```python
from build123d import *

# Parameters (mm, degrees)
F0_R     = 30
F1_DEPTH = 200
F5_START = 20
F4_R     = 45
F5_DEPTH = 30


with BuildPart() as f1:
    # F0 (on Right) → F1 (new body)
    with BuildSketch(Plane.YZ):
        Circle(F0_R)
    extrude(amount=-F1_DEPTH)

    # F2 (on Top) → F3 (revolve)
    with BuildSketch(Plane.XY):
        Polygon((0, 12.6511614473), (0, 0), (30.3976608496, 0), (30.3976608496, 8), align=None)
    revolve(axis=Axis((15.1988304248, 0, 0), (1, 0, 0)))

    # F4 (on Right) → F5 (join)
    with BuildSketch(Plane.YZ.offset(F5_START)):
        Circle(F4_R)
    extrude(amount=F5_DEPTH)


solid = f1.part
```
Read the model definition and answer for the solid it produces. Units are mm, in the model's axes. A direction names the side the tool comes from. Coordinates: 2 decimals unless noted, no trailing zeros. Loops run counter-clockwise (first coordinate to the right, second up) from the corner with the lowest first, then second, coordinate; pieces in that order, holes last.
(1) Consider line 1 along X through (y, z) = (25.5, 10); line 2 along X through (y, z) = (-4, -37.5); line 3 along Y through (x, z) = (-111, -0.5). Determine where each line is inside the solid, lowest interval first.
Solution:
line 1: x = -200 to 0, 20 to 50
line 2: x = 20 to 50
line 3: y = -30 to 30
(2) The part is cut by section A-A (y = 25). Determine the outline of the cut face in (x, z), and give its area (3 significant figures).
Solution:
outline: (-200, -16.58) - (0, -16.58) - (0, 16.58) - (-200, 16.58) - close; (20, -37.42) - (50, -37.42) - (50, 37.42) - (20, 37.42) - close
area: 8,880 mm2
(3) Flat-ended cylindrical pins translate along their axes: pin 1 Ø8 at (x, y) = (-128.5, 18) entering from -Z; pin 2 Ø1.5 at (x, y) = (-8, 2) entering from -Z; pin 3 Ø10 at (x, y) = (-12.5, -10) entering from -Z. Find the tip coordinate at first contact, or state that the pin passes through.
Solution:
pin 1: stops at z = -26.53
pin 2: stops at z = -29.97
pin 3: stops at z = -29.58
(4) The mould has two halves that part along X. Classify faces 1 (the face through (-200, 0, 0)), 2 (the face through (34.79, 20.765, -39.923)), 3 (the face through (0, 13, 0)): released by +X, released by -X, zero draft, split by the parting line, or undercut.
Solution:
face 1: released by -X
face 2: zero draft
face 3: undercut
(5) The part is cut by section D-D (y = 0). Determine the outline of the cut face in (x, z).
Solution:
outline: (-200, -30) - (0, -30) - (0, -12.65) - (20, -9.59) - (20, -45) - (50, -45) - (50, 45) - (20, 45) - (20, 9.59) - (0, 12.65) - (0, 30) - (-200, 30) - close
(6) The part is cut by section C-C (x = -146). Determine the outline of the cut face in (y, z), and give its area (3 significant figures).
Solution:
outline: circle Ø60 at (0, 0)
area: 2,830 mm2
(7) The part is cut by section B-B (z = 15). Determine the outline of the cut face in (x, y), and give its area (3 significant figures).
Solution:
outline: (-200, -25.98) - (0, -25.98) - (0, 25.98) - (-200, 25.98) - close; (20, -42.43) - (50, -42.43) - (50, 42.43) - (20, 42.43) - close
area: 12,900 mm2
(8) A tool of negligible diameter and unlimited length cuts with its end or side. For faces 4 (the face through (12.082, -2.342, -10.546)), 5 (the face through (50, -1, 1)), 6 (the face through (-98.6, -29.97, 1.32)), from which of +Z, -Z, +X, -X, +Y, -Y can it reach the whole face along a straight path? Write none if from no direction.
Solution:
face 4: none
face 5: +Z, -Z, +X, +Y, -Y
face 6: -X
